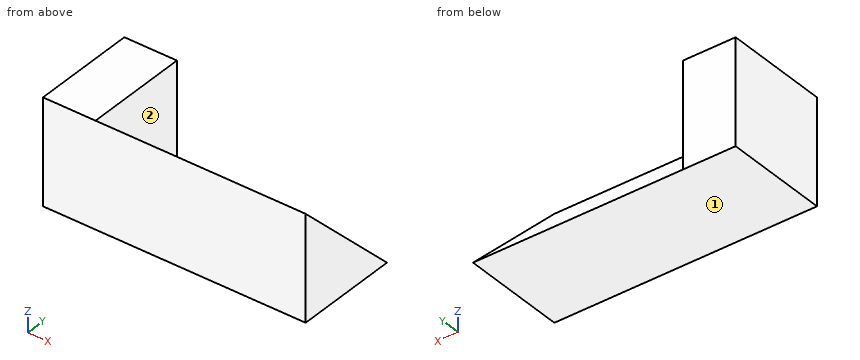
from build123d import *

# Parameters (mm, degrees)
F0_W     = 50
F0_H     = 20
F1_DEPTH = 20
F3_DEPTH = 40


with BuildPart() as f1:
    # F0 (on Top) → F1 (new body)
    with BuildSketch(Plane.XY):
        Rectangle(F0_W, F0_H)
    extrude(amount=F1_DEPTH)

    # F2 (on face) → F3 (cut)
    with BuildSketch(Plane.YZ.offset(25)):
        Polygon((10, 20), (-10, 20), (10, 0), align=None)
    extrude(amount=-F3_DEPTH, mode=Mode.SUBTRACT)


solid = f1.part
Read the model definition and answer for the solid it produces. Units are mm, in the model's axes. Face numbers are marked on the shaded views. A direction names the side the tool comes from. Coordinates: 2 decimals unless noted, no trailing zeros. Order: outer loops, then holes, each group sorted by start corner. A loop starts at its lowest first (then second) coordinate and runs counter-clockwise, first axis right, second up. Notation, with made-up numbers: (-33.5, 64.25) -> (17.5, 64.25) arc R36 cw to (17.5, 101.25) -> close; hole circle Ø10 at (36.25, 89). An arc over 180 degrees is marked (long way). Answer as a JSON object with one key per item and string values.
1) A cutting plane is placed at B-B, the plane y = 0.75. Determine the outline of the cut face in (x, z).
Model answer:
{"outline": "(-25, 0) -> (25, 0) -> (25, 9.25) -> (-15, 9.25) -> (-15, 20) -> (-25, 20) -> close"}
2) A cutting plane is placed at A-A, the plane z = 16.5. Determine the outline of the cut face in (x, y), plus the area to 3 significant figures.
Model answer:
{"outline": "(-25, -10) -> (25, -10) -> (25, -6.5) -> (-15, -6.5) -> (-15, 10) -> (-25, 10) -> close", "area": "340 mm²"}
3) A cutting plane is placed at C-C, the plane x = 11. Determine the outline of the cut face in (y, z), plus the area to 3 significant figures.
Model answer:
{"outline": "(-10, 0) -> (10, 0) -> (-10, 20) -> close", "area": "200 mm²"}
4) A tool of negligible diameter and unlimited length cuts with its end or side. For the marked faces 1 and 2, from which of +Z, -Z, +X, -X, +Y, -Y can it reach the whole face along a straight path? Write none if from no direction.
Model answer:
{"face 1": "-Z, +X, -X, +Y, -Y", "face 2": "+Z, +X, +Y"}
5) Each of these flat-tipped pins is pushed along its axis until it touches: pin 1 (8 mm diameter, centred on x = -2, y = -5.5, fed in from -Z); pin 2 (4 mm diameter, centred on x = 4, z = 12.5, fed in from +Y). Where does it stop, or does it pass through?
Model answer:
{"pin 1": "stops at z = 0", "pin 2": "stops at y = -0.5"}
6) Consider line 1 along X through (y, z) = (8.25, 14.5); line 2 along Z through (x, y) = (12.5, 0); line 3 along Y through (x, z) = (-3, 13). Determine where each line is inside the solid, lowest interval first. Write a range as from..to.
Model answer:
{"line 1": "x = -25..-15", "line 2": "z = 0..10", "line 3": "y = -10..-3"}
